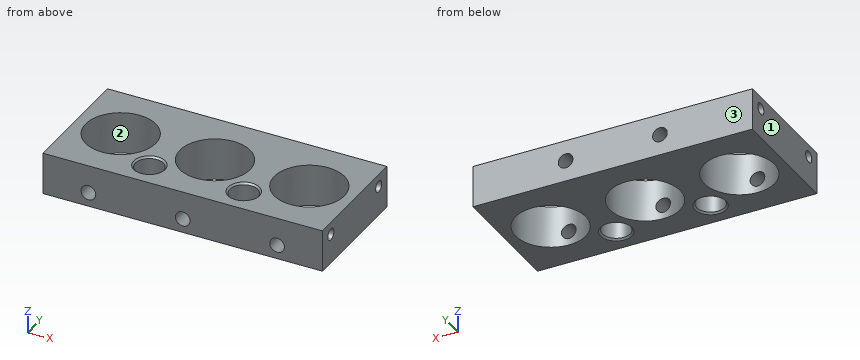
from build123d import *

# Parameters (mm, degrees)
F0_W      = 80
F0_H      = 35
F0_R      = 4
F0_R_2    = 10.05
F1_DEPTH  = 12
F2_SIZE   = 0.5
F3_R      = 2.1
F4_DEPTH  = 7.6728517519
F6_D      = 4.2
F6_DEPTH  = 15
F6_TIP    = 1.2618073
F8_D      = 3.3
F8_DEPTH  = 12
F8_TIP    = 0.9914200214
F10_D     = 3.3
F10_DEPTH = 12
F10_TIP   = 0.9914200214


with BuildPart() as f1:
    # F0 (on Top) → F1 (new body)
    with BuildSketch(Plane.XY):
        with Locations((40, 17.5)):
            Rectangle(F0_W, F0_H)
        with Locations((26.5, 7.5)):
            Circle(F0_R, mode=Mode.SUBTRACT)
        with Locations((53.5, 7.5)):
            Circle(F0_R, mode=Mode.SUBTRACT)
        with Locations((13, 17.5)):
            Circle(F0_R_2, mode=Mode.SUBTRACT)
        with Locations((40, 17.5)):
            Circle(F0_R_2, mode=Mode.SUBTRACT)
        with Locations((67, 17.5)):
            Circle(F0_R_2, mode=Mode.SUBTRACT)
    extrude(amount=F1_DEPTH)

    # F2
    f2_edges = [f1.edges().sort_by_distance(p)[0] for p in [
        (22.5, 7.5, 12),
        (49.5, 7.5, 12),
        (49.5, 7.5, 0),
        (22.5, 7.5, 0),
    ]]
    chamfer(f2_edges, length=F2_SIZE)

    # F3 (on face) → F4 (cut, through all)
    with BuildSketch(Plane.XZ):
        with Locations((40, 4)):
            Circle(F3_R)
        with Locations((67, 4)):
            Circle(F3_R)
        with Locations((13, 4)):
            Circle(F3_R)
    extrude(amount=-F4_DEPTH, mode=Mode.SUBTRACT)

    # F6
    with Locations(Plane(origin=(0, 35, 0), x_dir=(-1, 0, 0), z_dir=(0, 1, 0))):
        with Locations((-53.5, 6), (-26.5, 6)):
            Hole(F6_D / 2, depth=F6_DEPTH)
            with Locations((0, 0, -(F6_DEPTH + F6_TIP / 2))):  # 118° drill point
                Cone(0, F6_D / 2, F6_TIP, mode=Mode.SUBTRACT)

    # F8
    with Locations(Plane.YZ.offset(80)):
        with Locations((4.5, 8.5), (30.5, 8.5)):
            Hole(F8_D / 2, depth=F8_DEPTH)
            with Locations((0, 0, -(F8_DEPTH + F8_TIP / 2))):  # 118° drill point
                Cone(0, F8_D / 2, F8_TIP, mode=Mode.SUBTRACT)

    # F10
    with Locations(Plane(origin=(0, 0, 0), x_dir=(0, -1, 0), z_dir=(-1, 0, 0))):
        with Locations((-30.5, 8.5), (-4.5, 8.5)):
            Hole(F10_D / 2, depth=F10_DEPTH)
            with Locations((0, 0, -(F10_DEPTH + F10_TIP / 2))):  # 118° drill point
                Cone(0, F10_D / 2, F10_TIP, mode=Mode.SUBTRACT)


solid = f1.part
Build history of the part. All positions in model axes, mm. Face numbers are marked on the shaded views. Coordinates: 2 decimals unless noted, no trailing zeros. Order: outer loops, then holes, each group sorted by start corner. A loop starts at its lowest first (then second) coordinate and runs counter-clockwise, first axis right, second up. Notation, with made-up numbers: (-2.75, 42) - (28.25, 42) arc R35 cw to (28.25, 74) - close; hole circle Ø7 at (64.25, -35). An arc over 180 degrees is marked (long way). Write each question's results on one line, items separated by ' | '. Start each with the question number.
Item 1: Wall check: probe 1 along X at (y, z) = (3, 4); probe 2 along X at (y, z) = (18, 10.75); probe 3 along Y at (x, z) = (13, 10.25). Give the ranges that are in metal, low to high. Write a range as [from, to].
Item 2: Flat gauge pins, fed straight in: pin 1 (3 mm diameter, centred on y = 30.5, z = 8.5, fed in from +X); pin 2 (16 mm diameter, centred on x = 40, y = 17.5, fed in from -Z); pin 3 (2.5 mm diameter, centred on y = 30.5, z = 8.5, fed in from +X); pin 4 (3.5 mm diameter, centred on x = 26.5, z = 6, fed in from +Y). Where does each tip first touch, or does it go through?
Item 3: Mould opens along X. For the marked faces 1, 2 and 3 say: released by +X, released by -X, zero draft, split by the parting line, or undercut.
Item 4: Band-saw the part on C-C on y = 9. State how many separate pieces and enclosed holes the cut face has, and give its area (3 significant figures).
Item 5: Band-saw the part on B-B on x = 40. Write the cut outline in (y, z).
Item 6: Band-saw the part on A-A on y = 21. Write the cut outline in (x, z).
Numbers:
1) probe 1: [0, 10.9], [15.1, 37.9], [42.1, 64.9], [69.1, 80] | probe 2: [0, 2.96], [23.04, 29.96], [50.04, 56.96], [77.04, 80] | probe 3: [0, 7.45], [27.55, 35]
2) pin 1: x = 67.91 | pin 2: through | pin 3: x = 67.76 | pin 4: y = 19.79
3) face 1: released by -X | face 2: undercut | face 3: zero draft
4) separate pieces: 6 | enclosed holes: 0 | area: 395 mm^2
5) outline: (0, 0) - (7.45, 0) - (7.45, 1.9) - (0, 1.9) - close; (0, 6.1) - (7.45, 6.1) - (7.45, 12) - (0, 12) - close; (27.55, 0) - (35, 0) - (35, 12) - (27.55, 12) - close
6) outline: (0, 0) - (3.58, 0) - (3.58, 12) - (0, 12) - close; (22.42, 0) - (30.58, 0) - (30.58, 12) - (22.42, 12) - close; (49.42, 0) - (57.58, 0) - (57.58, 12) - (49.42, 12) - close; (76.42, 0) - (80, 0) - (80, 12) - (76.42, 12) - close; hole circle Ø4.2 at (26.5, 6); hole circle Ø4.2 at (53.5, 6)
